```python
from build123d import *

# Parameters (mm, degrees)
SKETCH1_W               = 40
SKETCH1_H               = 40
BOSS_EXTRUDE1_DEPTH     = 100
CUT_EXTRUDE1_DEPTH      = 104.923048454
CUT_EXTRUDE1_DEPTH_BACK = 104.923048454
SKETCH2_R               = 4


with BuildPart() as part:
    # Sketch1 → Boss-Extrude1 (new body)
    with BuildSketch(Plane(origin=(0, 0, 0), x_dir=(1, 0, 0), z_dir=(0, 1, 0))):
        Rectangle(SKETCH1_W, SKETCH1_H)
    extrude(amount=BOSS_EXTRUDE1_DEPTH)

    # Sketch2 → Cut-Extrude1 (cut, two sides: drawn at the far end of the back side and taken through both)
    with BuildSketch(Plane(origin=(0, 100, 0), x_dir=(1, 0, 0), z_dir=(0, 1, 0)).offset(-CUT_EXTRUDE1_DEPTH_BACK)):
        with Locations(Location((0, 0, 0), (0, 0, 270))):
            Circle(SKETCH2_R)
        Polygon((-7, 20), (-7, 18), (-12, 18), (-12, 14.121320344), (-5.878679656, 8), (5.878679656, 8), (12, 14.121320344), (12, 18), (7, 18), (7, 20), align=None)
        Polygon((20, 7), (18, 7), (18, 12), (14.121320344, 12), (8, 5.878679656), (8, -5.878679656), (14.121320344, -12), (18, -12), (18, -7), (20, -7), align=None)
        Polygon((7, -20), (7, -18), (12, -18), (12, -14.121320344), (5.878679656, -8), (-5.878679656, -8), (-12, -14.121320344), (-12, -18), (-7, -18), (-7, -20), align=None)
        Polygon((-20, -7), (-18, -7), (-18, -12), (-14.121320344, -12), (-8, -5.878679656), (-8, 5.878679656), (-14.121320344, 12), (-18, 12), (-18, 7), (-20, 7), align=None)
    extrude(amount=CUT_EXTRUDE1_DEPTH + CUT_EXTRUDE1_DEPTH_BACK, mode=Mode.SUBTRACT)


solid = part.part
```
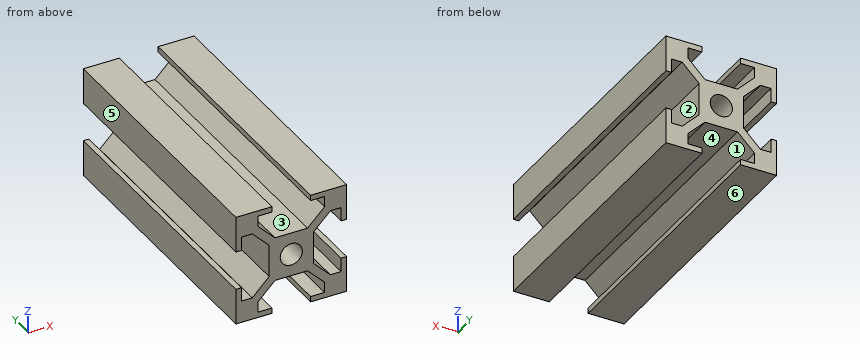
Source: CAD feature listing. Evaluate the final solid. Frame: model axes, mm. Face numbers are marked on the shaded views. A direction names the side the tool comes from. Give positions to 0.01 mm unless a question says otherwise; leave off trailing zeros. Write each loop counter-clockwise with the first axis right and the second up, starting at its lowest first coordinate (ties: lowest second). Pieces come first, ordered by that corner, then holes. Notation, with made-up numbers: (-10, -35) - (-4, -35) arc R21 ccw to (-4, -30) - close; hole circle Ø4 at (-18.75, -26.75). An arc over 180 degrees is marked (long way). One line per item, written item: value. Start each with the question number.
Q1. Section query B-B, the plane x = 0. Return the cut outline in (y, z).
Q2. Section query C-C, the plane x = 10.5. Return the cut outline in (y, z).
Q3. Material intervals for probe 1 along X at (y, z) = (33, 0); probe 2 along Z at (x, y) = (-14.5, 89), sorted ascending. Write a range as from..to.
Q4. Section query A-A, the plane z = 0. Return the cut outline in (x, y), then the cut area to 3 significant figures.
Q5. Draft query along X for the marked faces 4, 5 and 6. Return one class per face: +X half, -X half, draft (parallel to the pull), parting line (faces both ways), or undercut.
Q6. First-contact query: pin 1 Ø2 at (y, z) = (59.5, -5) entering from +X; pin 2 Ø1.5 at (x, z) = (-7, 12) entering from -Y; pin 3 Ø3 at (x, y) = (-3.5, 48.5) entering from -Z. Flat tips, straight axial feed; report the tip coordinate or a pass-through.
Q7. Set-up query: the marked faces 1, 2 and 3. Return all of +Z, -Z, +X, -X, +Y, -Y with unobstructed straight access to the full face (end or side cutting, diameter ignored); none if empty.
Answer:
1. outline: (0, -8) - (100, -8) - (100, -4) - (0, -4) - close; (0, 4) - (100, 4) - (100, 8) - (0, 8) - close
2. outline: (0, -20) - (100, -20) - (100, -18) - (0, -18) - close; (0, -12.62) - (100, -12.62) - (100, -8.38) - (0, -8.38) - close; (0, 8.38) - (100, 8.38) - (100, 12.62) - (0, 12.62) - close; (0, 18) - (100, 18) - (100, 20) - (0, 20) - close
3. probe 1: x = -8..-4, 4..8
3. probe 2: z = -20..-12, 12..20
4. outline: (-8, 0) - (-4, 0) - (-4, 100) - (-8, 100) - close; (4, 0) - (8, 0) - (8, 100) - (4, 100) - close
4. area: 800 mm2
5. face 4: undercut
5. face 5: -X half
5. face 6: draft
6. pin 1: stops at x = 8.12
6. pin 2: passes through
6. pin 3: stops at z = -8
7. face 1: +Y, -Y
7. face 2: +X, +Y, -Y
7. face 3: +Z, +Y, -Y
